```python
from build123d import *

# Parameters (mm, degrees)
SKETCH_1_R      = 31
SKETCH_1_R_2    = 17.5
EXTRUDE_1_DEPTH = 7
SKETCH_2_W      = 5.621005066
SKETCH_2_H      = 4.346885609


with BuildPart() as part:
    # 草图1 → 凸台-拉伸1 (new, symmetric)
    with BuildSketch(Plane.XY):
        Circle(SKETCH_1_R)
        Circle(SKETCH_1_R_2, mode=Mode.SUBTRACT)
    extrude(amount=EXTRUDE_1_DEPTH, both=True)

    # 草图2 → 切除-旋转1 (revolve, cut)
    with BuildSketch(Plane(origin=(0, 0, 0), x_dir=(1, 0, 0), z_dir=(0, 1, 0)), mode=Mode.PRIVATE) as cut_revolve_1_sk:
        with Locations((22.596440368, 4.826557196)):
            Rectangle(SKETCH_2_W, SKETCH_2_H)
    cut_revolve_1 = revolve(cut_revolve_1_sk.sketch.rotate(Axis((0, 0, -7), (0, 0, 1)), 180), axis=Axis((0, 0, -7), (0, 0, 1)), mode=Mode.SUBTRACT)

    # 镜向1: 切除-旋转1 across plane
    add(cut_revolve_1.mirror(Plane.XY), mode=Mode.SUBTRACT)


solid = part.part
```
Can you work these out from the model? Positions are in its coordinate system, mm. A direction names the side the tool comes from. Coordinates: 2 decimals unless noted, no trailing zeros. Loops run counter-clockwise (first coordinate to the right, second up) from the corner with the lowest first, then second, coordinate; pieces in that order, holes last. Notation, with made-up numbers: (-0.5, 78.5) -> (46.5, 78.5) arc R27 ccw to (46.5, 101.5) -> close; hole circle Ø3 at (42.5, 45.25). An arc over 180 degrees is marked (long way). Answer as a JSON object with one key per item and string values.
1) For faces 1 (the face through (12, -13, -7)), 2 (the face through (-18.872, -5.943, 4.857)), 3 (the face through (20.16, 15.46, -4.86)), which set-ups out of +Z, -Z, +X, -X, +Y, -Y let a thin tool reach every point of the face, with its end or its side?
Results:
{"face 1": "-Z, +X, -X, +Y, -Y", "face 2": "+Z", "face 3": "-Z"}
2) Imagine slicing it at D-D (x = 21.5). Please give me the cut outline in (y, z).
Results:
{"outline": "(-22.33, -7) -> (-13.54, -7) -> (-13.54, -2.65) -> (13.54, -2.65) -> (13.54, -7) -> (22.33, -7) -> (22.33, 7) -> (13.54, 7) -> (13.54, 2.65) -> (-13.54, 2.65) -> (-13.54, 7) -> (-22.33, 7) -> close"}
3) For P1, Ø3, axis at x = -14.5, z = 3, coming from the -Y side; P2, Ø6, axis at y = 24, z = -1, coming from the +X side; P3, Ø1, axis at x = -21, z = 3, coming from the +Y side; P4, Ø2, axis at x = -3, y = -15, coming from the +Z side, each with a flat end and sliding along its axis, tell me the tip position at first contact or that it passes through.
Results:
{"P1": "stops at y = -28.14", "P2": "stops at x = 22.8", "P3": "stops at y = 23.25", "P4": "passes through"}
4) Imagine slicing it at C-C (z = 0.75). Please give me the cut outline in (x, y).
Results:
{"outline": "circle Ø62 at (0, 0); hole circle Ø35 at (0, 0)"}
5) Thinking about a two-plate mould opening in X: for faces 4 (the face through (-4.036, 30.736, 0.098)), 5 (the face through (20.16, 15.46, 4.86)), 6 (the face through (4.4, 25.4, -7)), which applies, pulls with the +X half, pulls with the -X half, needs draft (parallel to the pull), parting line crosses it, or undercut?
Results:
{"face 4": "parting line crosses it", "face 5": "undercut", "face 6": "needs draft"}
6) If I drill on line 1 (Y direction, x = 0, z = 4.5); line 2 (Y direction, x = 0, z = 2); line 3 (X direction, y = 4, z = -5.5), over which ranges is the centre line in solid material (lowest first)?
Results:
{"line 1": "y = -31 to -25.41, -19.79 to -17.5, 17.5 to 19.79, 25.41 to 31", "line 2": "y = -31 to -17.5, 17.5 to 31", "line 3": "x = -30.74 to -25.09, -19.38 to -17.04, 17.04 to 19.38, 25.09 to 30.74"}
7) Imagine slicing it at A-A (y = 0). Please give me the cut outline in (x, z).
Results:
{"outline": "(-31, -7) -> (-25.41, -7) -> (-25.41, -2.65) -> (-19.79, -2.65) -> (-19.79, -7) -> (-17.5, -7) -> (-17.5, 7) -> (-19.79, 7) -> (-19.79, 2.65) -> (-25.41, 2.65) -> (-25.41, 7) -> (-31, 7) -> close; (17.5, -7) -> (19.79, -7) -> (19.79, -2.65) -> (25.41, -2.65) -> (25.41, -7) -> (31, -7) -> (31, 7) -> (25.41, 7) -> (25.41, 2.65) -> (19.79, 2.65) -> (19.79, 7) -> (17.5, 7) -> close"}
